Could you check a few things on this model? Use its own coordinates, in mm. A direction names the side the tool comes from. Give positions to 0.01 mm unless a question says otherwise; leave off trailing zeros. Order: outer loops, then holes, each group sorted by start corner. A loop starts at its lowest first (then second) coordinate and runs counter-clockwise, first axis right, second up. Notation, with made-up numbers: M -19,20.25 L 8,20.25 A9 ccw 8,33.25 Z; hole C 35,-14 d3. An arc over 180 degrees is marked long. Use a Markdown table: item, result. Add a question column.
Item 1: For faces 4 (the face through (0, -10, -5.5)), 5 (the face through (3, -2.8, 2)), 6 (the face through (1.3, 4, 3)), 7 (the face through (0, -9.8, 0)), which set-ups out of +Z, -Z, +X, -X, +Y, -Y let a thin tool reach every point of the face, with its end or its side?
Item 2: I'm going to push flat-ended pins straight in: pin 1 Ø1.2 at (x, y) = (1, -11.5) entering from +Z; pin 2 Ø1 at (x, z) = (-3, 2) entering from -Y; pin 3 Ø3 at (y, z) = (-7, 2.5) entering from +X; pin 4 Ø1.5 at (y, z) = (2.5, -5) entering from -X. Where does each tip first touch, or does it pass through?
Item 3: Suppose I cut it at A-A on z = -4.75. Write out the boundary of the cut face in (x, y).
Item 4: Suppose I cut it at C-C on z = 0.5. Write out the boundary of the cut face in (x, y).
Item 5: If we mould it in two halves opening along Z, with no side actions, what happens to faces 1 (the face through (0, -6.8, -3)), 2 (the face through (0, 7, -8)), 3 (the face through (0, 6, 5))? For each: released by +Z, released by -Z, zero draft, split by the parting line, or undercut.
Item 6: Suppose I cut it at D-D on x = -1. Write out the boundary of the cut face in (y, z).
Item 7: Suppose I cut it at B-B on x = 0. Write out the boundary of the cut face in (y, z).
Item 8: If I drill on L1, parallel to Z at x = -1.25, y = 5; L2, parallel to X at y = -7.5, z = 0.5; L3, parallel to Y at x = 1, z = -3.75, over which ranges is the centre line in solid material (lowest first)? Write a range as from..to.
from build123d import *

# Parameters (mm, degrees)
SZKIC1_W                    = 7.6
SZKIC1_H                    = 5.6
DODANIE_WYCI_GNI_CIE1_DEPTH = 5
SZKIC2_R                    = 2.3
SZKIC2_W                    = 2.6
SZKIC2_H                    = 1.8
DODANIE_WYCI_GNI_CIE2_DEPTH = 5
SZKIC3_W                    = 3.6
SZKIC3_H                    = 7
DODANIE_WYCI_GNI_CIE3_DEPTH = 5
SZKIC4_R                    = 2.3
DODANIE_WYCI_GNI_CIE4_DEPTH = 8
SFAZOWANIE1_SIZE            = 3
DODANIE_WYCI_GNI_CIE5_DEPTH = 7.6
DODANIE_WYCI_GNI_CIE6_DEPTH = 3.6


with BuildPart() as part:
    # Szkic1 → Dodanie-wyciągnięcie1 (new body)
    with BuildSketch(Plane.XY):
        Rectangle(SZKIC1_W, SZKIC1_H)
    extrude(amount=DODANIE_WYCI_GNI_CIE1_DEPTH)

    # Szkic2 → Dodanie-wyciągnięcie2 (add)
    with BuildSketch(Plane.XY.offset(5)):
        with Locations((0, 6.497366596)):
            Circle(SZKIC2_R)
        with Locations((0, 3.7)):
            Rectangle(SZKIC2_W, SZKIC2_H)
    extrude(amount=-DODANIE_WYCI_GNI_CIE2_DEPTH)

    # Szkic3 → Dodanie-wyciągnięcie3 (add)
    with BuildSketch(Plane.XY.offset(5)):
        with Locations((0, -6.3)):
            Rectangle(SZKIC3_W, SZKIC3_H)
    extrude(amount=-DODANIE_WYCI_GNI_CIE3_DEPTH)

    # Szkic4 → Dodanie-wyciągnięcie4 (add)
    with BuildSketch(Plane(origin=(0, 0, 0), x_dir=(-1, 0, 0), z_dir=(0, 0, -1))):
        with Locations(Location((0, 6.497366596, 0), (0, 0, 235.58261129))):
            Circle(SZKIC4_R)
    extrude(amount=DODANIE_WYCI_GNI_CIE4_DEPTH)

    # Sfazowanie1
    sfazowanie1_edges = [part.edges().sort_by_distance(p)[0] for p in [
        (0, -9.8, 5),
    ]]
    chamfer(sfazowanie1_edges, length=SFAZOWANIE1_SIZE)

    # Szkic5 → Dodanie-wyciągnięcie5 (add)
    with BuildSketch(Plane(origin=(3.8, 0, 0), x_dir=(0, 0, -1), z_dir=(1, 0, 0))):
        Polygon((-5, 2.8), (-8.5, 2.8), (-8.5, 1.8), (-5, -2.8), align=None)
    extrude(amount=-DODANIE_WYCI_GNI_CIE5_DEPTH)

    # Szkic6 → Dodanie-wyciągnięcie6 (add)
    with BuildSketch(Plane.ZY.offset(1.8)):
        Polygon((0, -9.8), (-3, -9.8), (-3, -12.3), (-5.5, -12.3), (-5.5, -6.8), (0, -6.8), align=None)
    extrude(amount=-DODANIE_WYCI_GNI_CIE6_DEPTH)


solid = part.part
Findings below:
| question | item | result |
|---|---|---|
| 1 | face 4 | -Z, +X, -X, -Y |
| 1 | face 5 | +Z, -Z, +X, -Y |
| 1 | face 6 | +Z, -Z, +X |
| 1 | face 7 | +Z, +X, -X, -Y |
| 2 | pin 1 | stops at z = -3 |
| 2 | pin 2 | stops at y = -2.8 |
| 2 | pin 3 | stops at x = 1.8 |
| 2 | pin 4 | passes through |
| 3 | outline | C 0,6.5 d4.6; M -1.8,-12.3 L 1.8,-12.3 L 1.8,-6.8 L -1.8,-6.8 Z |
| 4 | outline | M -3.8,-2.8 L -1.8,-2.8 L -1.8,-9.8 L 1.8,-9.8 L 1.8,-2.8 L 3.8,-2.8 L 3.8,2.8 L 1.3,2.8 L 1.3,4.6 A2.3 ccw long -1.3,4.6 L -1.3,2.8 L -3.8,2.8 Z |
| 5 | face 1 | zero draft |
| 5 | face 2 | released by -Z |
| 5 | face 3 | released by +Z |
| 6 | outline | M -12.3,-5.5 L -6.8,-5.5 L -6.8,0 L 4.43,0 L 4.43,-8 L 8.57,-8 L 8.57,5 L 2.8,5 L 2.8,8.5 L 1.8,8.5 L -2.8,5 L -6.8,5 L -9.8,2 L -9.8,-3 L -12.3,-3 Z |
| 7 | outline | M -12.3,-5.5 L -6.8,-5.5 L -6.8,0 L 4.2,0 L 4.2,-8 L 8.8,-8 L 8.8,5 L 2.8,5 L 2.8,8.5 L 1.8,8.5 L -2.8,5 L -6.8,5 L -9.8,2 L -9.8,-3 L -12.3,-3 Z |
| 8 | L1 | z = -8..5 |
| 8 | L2 | x = -1.8..1.8 |
| 8 | L3 | y = -12.3..-6.8, 4.43..8.57 |
